Autodesk Inventor part; units mm, degrees
ref_plane "YZ Plane" through (0, 0, 0) normal (1, 0, 0) x (0, 1, 0)
ref_plane "XZ Plane" through (0, 0, 0) normal (0, 1, 0) x (-1, 0, 0)
ref_plane "XY Plane" through (0, 0, 0) normal (0, 0, 1) x (1, 0, 0)
sketch "Sketch1" plane through (0, 0, 0) normal (0, 1, 0) x (-1, 0, 0)
  line L0 (35, 35) -> (35, 3)
  line L1 (9, 3) -> (35, 3) construction
  line L2 (0, 3) -> (9, 3) construction
  line L3 (35, 3) -> (50, 3)
  line L4 (0, -35) -> (0, 35)
  line L5 (0, -35) -> (50, -35)
  line L6 (0, 35) -> (35, 35)
  line L7 (50, -35) -> (50, 3)
  line L8 (30.7, 28.05) -> (35, 28.05) construction
  line L9 (30.7, 28.05) -> (30.7, 9.95) construction
  line L10 (30.7, 9.95) -> (30.7, 3) construction
  circle A0 centre (30.7, 9.95) radius 1.25
  circle A1 centre (30.7, 28.05) radius 1.25
  circle A2 centre (44, -3) radius 1.25
  arc A3 (0, -31.25) -> (0, -28.75) centre (0, -30) ccw
  arc A4 (0, 6.45) -> (0, 8.95) centre (0, 7.7) ccw
  arc A5 (0, 28.05) -> (0, 30.55) centre (0, 29.3) ccw
  line L11 (0, 29.3) -> (30.7, 29.3) construction
  line L12 (50, -35) -> (50, -65)
  line L13 (50, -65) -> (0, -65)
  line L14 (0, -35) -> (0, -65)
  circle A6 centre (44, -41) radius 1.25
  circle A7 centre (18, -41) radius 1.25
  circle A8 centre (18, -51) radius 1.25
  point P0 (0, 0)
  point P1 (-50, 0)
  point P2 (0, 0)
  dimension "d26" = 2.5
  dimension "d6" = 32
  dimension "d9" = 26
  dimension "d10" = 9
  dimension "d11" = 50
  dimension "d12" = 70
  dimension "d14" = 4.3
  dimension "d15" = 18.1
  dimension "d20" = 6.95
  dimension "d25" = 2.5
  dimension "d32" = 2.5
  dimension "d33" = 2.5
  dimension "d35" = 2.5
  dimension "d36" = 30
  dimension "d37" = 6
  dimension "d38" = 6
  dimension "d39" = 32
  dimension "d40" = 10
  dimension "d41" = 2.5
  dimension "d42" = 2.5
  dimension "d43" = 2.5
  dimension "d55" = 6
  dimension "d56" = 6
  dimension "d57" = 2.5
  dimension "d58" = 5
  dimension "d59" = 2.25
extrude "Extrusion1" add sketch "Sketch1" along normal blind 5 contours L0 L3 L7 L5 L4 A3 A4 A5 L6 | A5 L4 | L12 L13 L14 L5 | A4 L4 | L4 A3 | A0 | A1 | A2
extrude "Extrusion4" cut sketch "Sketch1" along normal through all contours A5 L4 | A4 L4 | L4 A3 | A0 | A1 | A2
mirror "Mirror1" about plane through (0, 0, 0) normal (1, 0, 0) of "Extrusion1", "Extrusion4"
sketch "Sketch4" plane through (-50, 0, -65) normal (-1, 0, 0) x (0, 0, 1)
  line L0 (0, 5) -> (68, 5)
  line L1 (0, 5) -> (5, 5)
  line L2 (0, 0) -> (68, 0)
  line L3 (5, 5) -> (0, 0)
  line L4 (0, 0) -> (0, 5)
  line L5 (0, 0) -> (0, 5)
  point P0 (65, 0)
  dimension "d44" = 5
extrude "Extrusion5" cut sketch "Sketch4" against normal through all
sketch "Sketch5" plane through (0, 5, 0) normal (0, 1, 0) x (1, 0, 0)
  circle A0 centre (-40, 49) radius 6
  line L0 (-50, 60) -> (-50, -3)
  line L1 (50, 60) -> (-50, 60)
  point P0 (0, 0)
  dimension "d50" = 10
  dimension "d51" = 11
  dimension "d52" = 12
extrude "Extrusion6" cut sketch "Sketch5" against normal through all
mirror "Mirror2" about plane through (0, 0, 0) normal (1, 0, 0) of "Extrusion6"
properties part number "Podstawa_All_in_One_5mm"
Could you check a few things on this model? Use its own coordinates, in mm. A direction names the side the tool comes from. Give positions to 0.01 mm unless a question says otherwise; leave off trailing zeros. Order: outer loops, then holes, each group sorted by start corner. A loop starts at its lowest first (then second) coordinate and runs counter-clockwise, first axis right, second up.
Item 1: For faces 4 (the face through (-35, 2, 19)), 5 (the face through (43, 2, 3)), 6 (the face through (17.84, 2.46, -49.76)), which set-ups out of +Z, -Z, +X, -X, +Y, -Y let a thin tool reach every point of the face, with its end or its side?
Item 2: If we section it at C-C, the plane y = 1.75: Count the separate pieces of the cut face and the enclosed holes in it, plus the area to 3 significant figures.
Item 3: If we section it at D-D, the plane x = 18: Write out the boundary of the cut face in (y, z), plus the area to 4 significant figures.
Item 4: If we mould it in two halves opening along X, with no side actions, what happens to faces 1 (the face through (0.05, 2.46, 8.95)), 2 (the face through (1, 0, -14)), 3 (the face through (50, 2, -31))? For each: pulls with the +X half, pulls with the -X half, needs draft (parallel to the pull), parting line crosses it, or undercut.
Item 5: If we section it at B-B, the plane z = -41: Write out the boundary of the cut face in (x, y), plus the area to 3 significant figures.
Item 6: I'm going to push flat-ended pins straight in: pin 1 (2 mm diameter, centred on x = 0, z = 7.7, fed in from +Y); pin 2 (14 mm diameter, centred on x = -40, z = -49, fed in from -Y); pin 3 (1 mm diameter, centred on y = 1.5, z = 6.5, fed in from +X). Where does each tip first touch, or does it pass through?
Item 7: I need wall thicknesses on line 1 (X direction, y = 4.6, z = -49); line 2 (Z direction, x = 18.5, y = 0.8); line 3 (X direction, y = 4.3, z = -50.5). Which ranges of each line are inside material? Lowest first, please.
Item 8: If we section it at A-A, the plane x = 40: Write out the boundary of the cut face in (y, z), plus the area to 4 significant figures.
Values:
1. face 4: +Z, -X, +Y, -Y
1. face 5: +Z, +X, +Y, -Y
1. face 6: +Y, -Y
2. separate pieces: 1
2. enclosed holes: 17
2. area: 8,570 mm2
3. outline: (0, -65) - (5, -60) - (5, -52.25) - (0, -52.25) - close; (0, -49.75) - (5, -49.75) - (5, -42.25) - (0, -42.25) - close; (0, -39.75) - (5, -39.75) - (5, 35) - (0, 35) - close
3. area: 462.5 mm2
4. face 1: undercut
4. face 2: needs draft
4. face 3: pulls with the +X half
5. outline: (-50, 0) - (-45.25, 0) - (-45.25, 5) - (-50, 5) - close; (-42.75, 0) - (-19.25, 0) - (-19.25, 5) - (-42.75, 5) - close; (-16.75, 0) - (16.75, 0) - (16.75, 5) - (-16.75, 5) - close; (19.25, 0) - (42.75, 0) - (42.75, 5) - (19.25, 5) - close; (45.25, 0) - (50, 0) - (50, 5) - (45.25, 5) - close
5. area: 450 mm2
6. pin 1: passes through
6. pin 2: stops at y = 0
6. pin 3: stops at x = 35
7. line 1: x = -50 to -46, -34 to 34, 46 to 50
7. line 2: z = -64.2 to -52.15, -49.85 to -42.15, -39.85 to 35
7. line 3: x = -50 to -45.81, -34.19 to -19.15, -16.85 to 16.85, 19.15 to 34.19, 45.81 to 50
8. outline: (0, -65) - (5, -60) - (5, -55) - (0, -55) - close; (0, -43) - (5, -43) - (5, 3) - (0, 3) - close
8. area: 267.5 mm2
